from build123d import *

# Parameters (mm, degrees)
STOCK_BASE_SKEWED_1_OUTLINE_R = 0.95
STOCK_BASE_SKEWED_1_DEPTH     = 1.1
STOCK_BASE_SKEWED_1_START     = 1.1
STOCK_BASE_SKEWED_1_2_DEPTH   = 5.8
SKETCH1_W                     = 5.8
SKETCH1_H                     = 0.6
CUT_EXTRUDE1_DEPTH            = 18.76345965


# Read off the part's stored shape, not the designer's step: Stock-Base_skewed-1
with BuildPart() as part:
    # Stock-Base_skewed-1 outline → Stock-Base_skewed-1 (new body)
    with BuildSketch(Plane.XY):
        with BuildLine():
            Line((8.949972222, -0.011666667), (8.999971655, 10.488095238))
            ThreePointArc((8.999971655, 10.488095238), (7.184905048, 12.904351279), (4.369026688, 11.807269193))
            Line((4.369026688, 11.807269193), (-2.088353846, 1.281123809))
            ThreePointArc((-2.088353846, 1.281123809), (-2.417250501, -0.399249317), (-1.565479113, -1.884615385))
            ThreePointArc((-1.565479113, -1.884615385), (-1.415835135, -1.970269972), (-1.245993579, -2))
            Line((-1.245993579, -2), (-1.245993579, -7))
            Line((-1.245993579, -7), (7.745993579, -7))
            Line((7.745993579, -7), (7.745993579, -2))
            ThreePointArc((7.745993579, -2), (7.915835135, -1.970269972), (8.065479113, -1.884615385))
            ThreePointArc((8.065479113, -1.884615385), (8.715388585, -1.046209071), (8.949972222, -0.011666667))
        make_face()
        with BuildLine():
            ThreePointArc((7.463119607, 2.75282442), (7.325518036, 2.467571215), (7.017292273, 2.394766941))
            ThreePointArc((7.017292273, 2.394766941), (4.297058288, 1.072169676), (4.934520887, -1.884615385))
            ThreePointArc((4.934520887, -1.884615385), (5.084164865, -1.970269972), (5.254006421, -2))
            Line((5.254006421, -2), (1.245993579, -2))
            ThreePointArc((1.245993579, -2), (1.415835135, -1.970269972), (1.565479113, -1.884615385))
            ThreePointArc((1.565479113, -1.884615385), (2.412392059, 0.427626653), (0.822306837, 2.307880297))
            ThreePointArc((0.822306837, 2.307880297), (0.598713954, 2.532178772), (0.632085047, 2.847123137))
            Line((0.632085047, 2.847123137), (4.449478669, 9.069838376))
            ThreePointArc((4.449478669, 9.069838376), (5.815094952, 8.095648721), (7.489077768, 8.203976226))
            Line((7.489077768, 8.203976226), (7.463119607, 2.75282442))
        make_face(mode=Mode.SUBTRACT)
        Circle(STOCK_BASE_SKEWED_1_OUTLINE_R, mode=Mode.SUBTRACT)
        with Locations((6.5, 0)):
            Circle(STOCK_BASE_SKEWED_1_OUTLINE_R, mode=Mode.SUBTRACT)
        with Locations((6.5, 10.5)):
            Circle(STOCK_BASE_SKEWED_1_OUTLINE_R, mode=Mode.SUBTRACT)
    extrude(amount=STOCK_BASE_SKEWED_1_DEPTH)

    # Stock-Base_skewed-1 2 outline → Stock-Base_skewed-1 2 (add)
    with BuildSketch(Plane.XY.offset(STOCK_BASE_SKEWED_1_START)):
        with BuildLine():
            Line((7.487534665, 7.879928382), (7.481545884, 6.622298661))
            ThreePointArc((7.481545884, 6.622298661), (8.272723591, 6.914271194), (8.985102612, 7.365631642))
            Line((8.985102612, 7.365631642), (8.990799579, 8.561981048))
            ThreePointArc((8.990799579, 8.561981048), (8.86000918, 8.750577627), (8.638081723, 8.6920712))
            ThreePointArc((8.638081723, 8.6920712), (8.114702276, 8.212482446), (7.487534665, 7.879928382))
        make_face()
        with BuildLine():
            Line((3.762240232, 7.94957426), (4.280029642, 8.793620321))
            ThreePointArc((4.280029642, 8.793620321), (3.922249334, 9.406747282), (3.73015902, 10.090145211))
            ThreePointArc((3.73015902, 10.090145211), (3.572375767, 10.256816274), (3.361835371, 10.165451404))
            Line((3.361835371, 10.165451404), (2.736247989, 9.14568438))
            ThreePointArc((2.736247989, 9.14568438), (3.033358957, 8.50440488), (3.438697229, 7.925427153))
            ThreePointArc((3.438697229, 7.925427153), (3.606647644, 7.854710493), (3.762240232, 7.94957426))
        make_face()
    extrude(amount=STOCK_BASE_SKEWED_1_2_DEPTH)

    # Sketch1 → Cut-Extrude1 (cut, through all)
    with BuildSketch(Plane(origin=(7.449841837, -0.03547584, 0), x_dir=(0, 0, 1), z_dir=(-0.999988662067245, 0.004761904761905177, 0))):
        with Locations((4, 6.957849986)):
            Rectangle(SKETCH1_W, SKETCH1_H)
    extrude(amount=-CUT_EXTRUDE1_DEPTH, mode=Mode.SUBTRACT)


solid = part.part
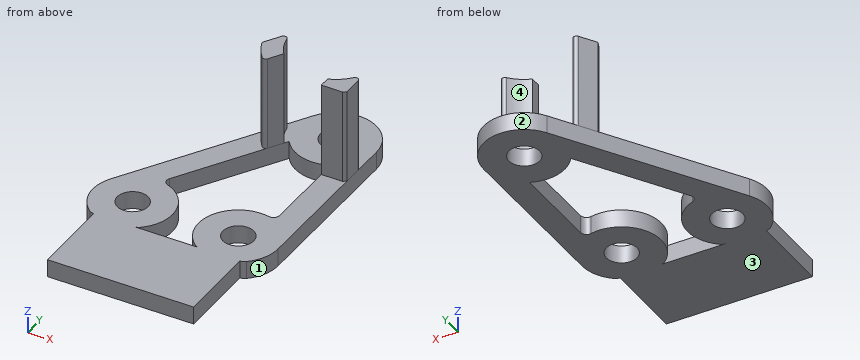
Can you work these out from the model? Positions are in its coordinate system, mm. Face numbers are marked on the shaded views. Round coordinates to 2 decimals unless told otherwise and drop trailing zeros. Write each loop counter-clockwise with the first axis right and the second up, starting at its lowest first coordinate (ties: lowest second). Pieces come first, ordered by that corner, then holes. Notation, with made-up numbers: M 20.25,-31 L 76.25,-31 A9 ccw 76.25,-24 Z; hole C -18,83 d3. An arc over 180 degrees is marked long. Use CSV: the item, a comma, the result in double quotes.
(1) Imagine slicing it at B-B (x = 6). Write out the boundary of the cut face in (y, z), plus the area to 3 significant figures.
Check values:
outline,"M -7,0 L -0.81,0 L -0.81,1.1 L -7,1.1 Z; M 0.81,0 L 2.4,0 L 2.4,1.1 L 0.81,1.1 Z; M 8.05,0 L 9.69,0 L 9.69,1.1 L 8.05,1.1 Z; M 11.31,0 L 12.95,0 L 12.95,1.1 L 11.31,1.1 Z"
area,"12.2 mm^2"
(2) We'd pull the mould along X, two halves only. Please class the marked faces 1, 2, 3 and 4: +X half, -X half, draft (parallel to the pull), parting line (faces both ways), or undercut.
Check values:
face 1,"+X half"
face 2,"parting line"
face 3,"draft"
face 4,"undercut"
(3) Imagine slicing it at C-C (z = 0.5). Write out the boundary of the cut face in (x, y), plus the area to 3 significant figures.
Check values:
outline,"M -2.09,1.28 A2.45 ccw -1.57,-1.88 A0.5 ccw -1.25,-2 L -1.25,-7 L 7.75,-7 L 7.75,-2 A0.5 ccw 8.07,-1.88 A2.45 ccw 8.95,-0.01 L 9,10.49 A2.5 ccw 4.37,11.81 Z; hole C 0,0 d1.9; hole M 0.63,2.85 A0.37 ccw 0.82,2.31 A2.45 cw 1.57,-1.88 A0.5 cw 1.25,-2 L 5.25,-2 A0.5 cw 4.93,-1.88 A2.45 cw 7.02,2.39 A0.37 ccw 7.46,2.75 L 7.49,8.2 A2.5 cw 4.45,9.07 Z; hole C 6.5,0 d1.9; hole C 6.5,10.5 d1.9"
area,"117 mm^2"
(4) Imagine slicing it at A-A (z = 6). Write out the boundary of the cut face in (x, y), plus the area to 3 significant figures.
Check values:
outline,"M 2.74,9.15 A4 ccw 3.44,7.93 A0.2 ccw 3.76,7.95 L 4.28,8.79 A2.8 cw 3.73,10.09 A0.2 ccw 3.36,10.17 Z; M 7.48,7.22 L 8.78,7.22 A4 ccw 8.99,7.37 L 8.99,8.56 A0.2 ccw 8.64,8.69 A2.8 cw 7.49,7.88 Z"
area,"3.75 mm^2"
(5) I'm going to push flat-ended pins straight in: pin 1 (0.6 mm diameter, centred on y = -5, z = 0.5, fed in from -X); pin 2 (2 mm diameter, centred on y = 9, z = 6, fed in from +X); pin 3 (4 mm diameter, centred on x = 6, y = 10, fed in from +Z). Where does each tip first touch, or does it pass through?
Check values:
pin 1,"x = -1.25"
pin 2,"x = 8.99"
pin 3,"z = 1.1"
(6) I need wall thicknesses on line 1 along Y through (x, z) = (6.5, 0.85); line 2 along Y through (x, z) = (1.75, 0.75); line 3 along Z through (x, y) = (4.5, 9.5). Which ranges of each line are inside material? Lowest first, please.
Check values:
line 1,"-7 to -0.95, 0.95 to 2.45, 8 to 9.55, 11.45 to 13"
line 2,"-7 to -2, -1.71 to 1.71, 4.67 to 7.54"
line 3,"0 to 1.1"
(7) Imagine slicing it at D-D (x = 0). Write out the boundary of the cut face in (y, z), plus the area to 3 significant figures.
Check values:
outline,"M -7,0 L -0.95,0 L -0.95,1.1 L -7,1.1 Z; M 0.95,0 L 4.69,0 L 4.69,1.1 L 0.95,1.1 Z"
area,"10.8 mm^2"
